Input: part model. Units: mm. Frame: model coordinates. Face numbers are marked on the shaded views. A direction names the side the tool comes from. Coordinates: 2 decimals unless noted, no trailing zeros. Loops run counter-clockwise (first coordinate to the right, second up) from the corner with the lowest first, then second, coordinate; pieces in that order, holes last.
```python
from build123d import *

# Parameters (mm, degrees)
PAD_DEPTH         = 30
PAD001_DEPTH      = 60
POCKET_DEPTH      = 30.001
POCKET_DEPTH_BACK = -30.001
SKETCH003_W       = 20
SKETCH003_H       = 20
POCKET001_DEPTH   = 60.001


with BuildPart() as part:
    # Sketch → Pad (new body, symmetric)
    with BuildSketch(Plane.XZ):
        Polygon((0, 30), (0, 0), (50, 0), (50, 60), (30, 60), align=None)
    extrude(amount=PAD_DEPTH, both=True)

    # Sketch001 → Pad001 (join)
    with BuildSketch(Plane.XY):
        Polygon((50, 30), (50, -30), (80, -20), (80, 20), align=None)
    extrude(amount=PAD001_DEPTH)

    # Sketch002 → Pocket (cut, two sides)
    with BuildSketch(Plane.XZ) as pocket_sk:
        Polygon((80, 50), (80, 10), (50, 30), align=None)
    extrude(amount=-POCKET_DEPTH, mode=Mode.SUBTRACT)
    extrude(pocket_sk.sketch, amount=-POCKET_DEPTH_BACK, mode=Mode.SUBTRACT)

    # Sketch003 → Pocket001 (cut, through all)
    with BuildSketch(Plane.XY):
        with Locations((10, 0)):
            Rectangle(SKETCH003_W, SKETCH003_H)
    extrude(amount=POCKET001_DEPTH, mode=Mode.SUBTRACT)


solid = part.part
```
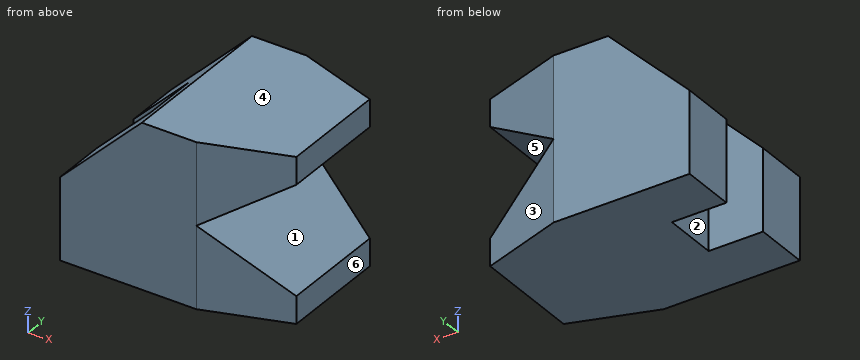
Item 1: Section query A-A (x = 65). Output: boundary loops of the cut face in (y, z).
Result:
outline: (-25, 0) - (25, 0) - (25, 20) - (-25, 20) - close; (-25, 40) - (25, 40) - (25, 60) - (-25, 60) - close
Item 2: Section query C-C (z = 4). Output: boundary loops of the cut face in (x, y).
Result:
outline: (0, -30) - (50, -30) - (80, -20) - (80, 20) - (50, 30) - (0, 30) - (0, 10) - (20, 10) - (20, -10) - (0, -10) - close
Item 3: Section query B-B (y = 3). Output: boundary loops of the cut face in (x, z), then the cut area to 3 significant figures.
Result:
outline: (20, 0) - (80, 0) - (80, 10) - (50, 30) - (80, 50) - (80, 60) - (30, 60) - (20, 50) - close
area: 2,950 mm2
Item 4: Reachability of the marked faces 1, 2 and 3 from +Z, -Z, +X, -X, +Y, -Y: full face, straight path, thin tool, end or side. Return the list, or none.
Result:
face 1: +X, +Y, -Y
face 2: +Z, -Z, -X
face 3: +Z, -Z, +X, +Y
Item 5: Line query: L1, parallel to Y at x = 17, z = 17; L2, parallel to Z at x = 57.5, y = -11; L3, parallel to Z at x = 54.5, y = -6. Output: solid intervals per line, ascending.
Result:
L1: y = -30 to -10, 10 to 30
L2: z = 0 to 25, 35 to 60
L3: z = 0 to 27, 33 to 60
Item 6: Contact query for flat-ended pins moving along their axis: P1, Ø6, axis at y = -2, z = 46.5, coming from the -X side; P2, Ø1, axis at x = 66.5, z = 42, coming from the +Y side. Output: stop coordinate, or through.
Result:
P1: stops at x = 20
P2: stops at y = 24.67
Item 7: Mould query, pull axis Z, two halves, no side actions, for the marked faces 4, 5 and 6. Classes: +Z half, -Z half, draft (parallel to the pull), parting line (faces both ways), or undercut.
Result:
face 4: +Z half
face 5: undercut
face 6: draft
Item 8: Section query D-D (z = 14.5). Output: boundary loops of the cut face in (x, y).
Result:
outline: (0, -30) - (50, -30) - (73.25, -22.25) - (73.25, 22.25) - (50, 30) - (0, 30) - (0, 10) - (20, 10) - (20, -10) - (0, -10) - close
